Geometry: final body of the model. Coordinates: model frame, mm. A direction names the side the tool comes from. Give positions to 0.01 mm unless a question says otherwise; leave off trailing zeros. Order: outer loops, then holes, each group sorted by start corner. A loop starts at its lowest first (then second) coordinate and runs counter-clockwise, first axis right, second up. Notation, with made-up numbers: (1.5, -32.5) -> (26.5, -32.5) arc R10 ccw to (26.5, -17.5) -> close; hole circle Ø2 at (23, 39.25). An arc over 180 degrees is marked (long way). One line per question, with ' | ' between items.
from build123d import *

# Parameters (mm, degrees)
F1_DEPTH = 10
F2_R     = 3.084409
F2_R_2   = 3.349591
F3_DEPTH = 2


with BuildPart() as f1:
    # F0 (on Front) → F1 (new body)
    with BuildSketch(Plane.XZ):
        Polygon((-25.699907, 57.854638), (-61.035037, 22.479102), (9.716036, -48.191159), (16.436929, -40.786458), (-46.900976, 22.479102), (-18.624799, 50.787612), align=None)
    extrude(amount=F1_DEPTH)

    # F2 (on face) → F3 (join)
    with BuildSketch(Plane(origin=(0, 0, 0), x_dir=(-1, 0, 0), z_dir=(0, 1, 0))):
        with Locations((-7.014304, -38.225602)):
            Circle(F2_R)
        with Locations((32.67004, 43.702345)):
            Circle(F2_R_2)
    extrude(amount=F3_DEPTH)


solid = f1.part
1) Section C-C on x = 5. Return loops of the section in (y, z).
Check result:
outline: (-10, -43.48) -> (0, -43.48) -> (0, -40.56) -> (2, -40.56) -> (2, -35.89) -> (0, -35.89) -> (0, -29.36) -> (-10, -29.36) -> close
2) Material intervals for probe 1 along Y at (x, z) = (-53.5, 20.5); probe 2 along Z at (x, y) = (-39, -3.5); probe 3 along Z at (x, y) = (-43.5, -8), sorted ascending. Write a range as from..to.
Check result:
probe 1: y = -10..0 | probe 2: z = 0.47..14.59, 30.39..44.54 | probe 3: z = 4.96..19.08, 25.88..40.03
3) Section A-A on x = -22. Return loops of the section in (y, z), plus the area to 3 significant figures.
Check result:
outline: (-10, -16.51) -> (0, -16.51) -> (0, -2.39) -> (-10, -2.39) -> close; (-10, 47.41) -> (0, 47.41) -> (0, 54.16) -> (-10, 54.16) -> close | area: 209 mm^2
4) Section B-B on y = -5.25. Return loops of the section in (x, z).
Check result:
outline: (-61.04, 22.48) -> (9.72, -48.19) -> (16.44, -40.79) -> (-46.9, 22.48) -> (-18.62, 50.79) -> (-25.7, 57.85) -> close
5) Contact query for flat-ended pins moving along their axis: pin 1 Ø4 at (x, y) = (-32.5, -3) entering from -Z; pin 2 Ø23 at (x, z) = (-30, 17.5) entering from +Y; pin 3 Ø1 at (x, y) = (-45.5, 0) entering from -Z; pin 4 Ø10 at (x, z) = (-26, -21) entering from -Y (3 decimals). Output: stop coordinate, or through.
Check result:
pin 1: stops at z = -8.02 | pin 2: stops at y = 0 | pin 3: stops at z = 6.46 | pin 4: passes through
6) Set-up query: faces 1 (the flat face through (-32.961, -4.93, 36.435)), 2 (the flat face through (-22.11, -4.93, 54.27)), 3 (the cylindrical face through (7.42, 0.99, -35.17)). Return all of +Z, -Z, +X, -X, +Y, -Y with unobstructed straight access to the full face (end or side cutting, diameter ignored); none if empty.
Check result:
face 1: +X, +Y, -Y | face 2: +Z, +X, +Y, -Y | face 3: +Y
7) Section D-D on z = -32.5. Return loops of the section in (x, y).
Check result:
outline: (-5.99, -10) -> (8.14, -10) -> (8.14, 0) -> (-5.99, 0) -> close
